```python
from build123d import *
from OCP.BRepFilletAPI import BRepFilletAPI_MakeChamfer

# Parameters (mm, degrees)
SM_BASE_FLANGE_1_DEPTH = 120
CUT_EXTRUDE_1_REACH    = 139.391
SKETCH_6_R             = 1.6
CHAMFER_1_SIZE         = 10
CHAMFER_1_SIZE2        = 50
SKETCH_7_R             = 2.7
CUT_EXTRUDE_2_DEPTH    = 2
SKETCH_9_R             = 2.1
CUT_EXTRUDE_3_DEPTH    = 2
CHAMFER_2_SIZE         = 40
CHAMFER_2_SIZE2        = 15
FILLET_1_R             = 5


# Sheet-metal steps are written as plain solids
with BuildPart() as part:
    # Sketch 1 → 基材-凸緣1 (new body)
    with BuildSketch(Plane.XY):
        with BuildLine():
            Line((-30, 17.5), (-30, -16))
            ThreePointArc((-30, -16), (-29.560660172, -17.060660172), (-28.5, -17.5))
            Line((-28.5, -17.5), (28.5, -17.5))
            ThreePointArc((28.5, -17.5), (29.560660172, -17.060660172), (30, -16))
            Line((30, -16), (30, 17.5))
            Line((30, 17.5), (32, 17.5))
            Line((32, 17.5), (32, -16))
            ThreePointArc((32, -16), (30.974873734, -18.474873734), (28.5, -19.5))
            Line((28.5, -19.5), (-28.5, -19.5))
            ThreePointArc((-28.5, -19.5), (-30.974873734, -18.474873734), (-32, -16))
            Line((-32, -16), (-32, 17.5))
            Line((-32, 17.5), (-30, 17.5))
        make_face()
    extrude(amount=SM_BASE_FLANGE_1_DEPTH)

    # 草圖6 → 除料-伸長1 (cut, up to next)
    with BuildSketch(Plane(origin=(32, 0, 0), x_dir=(0, 0, -1), z_dir=(1, 0, 0)), mode=Mode.PRIVATE) as cut_extrude_1_sk1:
        with Locations(Location((-107.5, 3.5, 0), (0, 0, 90))):
            Circle(SKETCH_6_R)
    cut_extrude_1_tool1 = extrude(cut_extrude_1_sk1.sketch, amount=-CUT_EXTRUDE_1_REACH, mode=Mode.PRIVATE) & part.part
    # 草圖6 → 除料-伸長1 (cut, up to next)
    with BuildSketch(Plane(origin=(32, 0, 0), x_dir=(0, 0, -1), z_dir=(1, 0, 0)), mode=Mode.PRIVATE) as cut_extrude_1_sk2:
        with Locations(Location((-100.5, -3.5, 0), (0, 0, 90))):
            Circle(SKETCH_6_R)
    cut_extrude_1_tool2 = extrude(cut_extrude_1_sk2.sketch, amount=-CUT_EXTRUDE_1_REACH, mode=Mode.PRIVATE) & part.part
    # 草圖6 → 除料-伸長1 (cut, up to next)
    with BuildSketch(Plane(origin=(32, 0, 0), x_dir=(0, 0, -1), z_dir=(1, 0, 0)), mode=Mode.PRIVATE) as cut_extrude_1_sk3:
        with Locations(Location((-107.5, -10.5, 0), (0, 0, 90))):
            Circle(SKETCH_6_R)
    cut_extrude_1_tool3 = extrude(cut_extrude_1_sk3.sketch, amount=-CUT_EXTRUDE_1_REACH, mode=Mode.PRIVATE) & part.part
    # 草圖6 → 除料-伸長1 (cut, up to next)
    with BuildSketch(Plane(origin=(32, 0, 0), x_dir=(0, 0, -1), z_dir=(1, 0, 0)), mode=Mode.PRIVATE) as cut_extrude_1_sk4:
        with Locations(Location((-114.5, -3.5, 0), (0, 0, 90))):
            Circle(SKETCH_6_R)
    cut_extrude_1_tool4 = extrude(cut_extrude_1_sk4.sketch, amount=-CUT_EXTRUDE_1_REACH, mode=Mode.PRIVATE) & part.part
    add(cut_extrude_1_tool1.solids().sort_by_distance((32, 3.5, 107.5))[0], mode=Mode.SUBTRACT)
    add(cut_extrude_1_tool2.solids().sort_by_distance((32, -3.5, 100.5))[0], mode=Mode.SUBTRACT)
    add(cut_extrude_1_tool3.solids().sort_by_distance((32, -10.5, 107.5))[0], mode=Mode.SUBTRACT)
    add(cut_extrude_1_tool4.solids().sort_by_distance((32, -3.5, 114.5))[0], mode=Mode.SUBTRACT)

    # 導角1
    chamfer_1_edges = [part.edges().sort_by_distance(p)[0] for p in [
        (-31, 17.5, 120),
        (31, 17.5, 120),
    ]]
    chamfer_1_side = [part.faces().sort_by_distance(p)[0] for p in [
        (-30.452140533, -17.952140533, 120),
    ]]
    chamfer(chamfer_1_edges, length=CHAMFER_1_SIZE, length2=CHAMFER_1_SIZE2, reference=chamfer_1_side[0])

    # 草圖7 → 除料-伸長2 (cut)
    with BuildSketch(Plane(origin=(32, 0, 0), x_dir=(0, 0, -1), z_dir=(1, 0, 0))):
        with Locations(Location((-107.5, -3.5, 0), (0, 0, 90))):
            Circle(SKETCH_7_R)
    extrude(amount=-CUT_EXTRUDE_2_DEPTH, mode=Mode.SUBTRACT)

    # 草圖9 → 除料-伸長3 (cut)
    with BuildSketch(Plane.ZY.offset(32)):
        with Locations(Location((107.5, -3.5, 0), (0, 0, 270))):
            Circle(SKETCH_9_R)
    extrude(amount=-CUT_EXTRUDE_3_DEPTH, mode=Mode.SUBTRACT)

    # 導角2: one chamfer whose edges measure the first distance from different faces: ONE call of the kernel's chamfer builder (chamfer() names one face for all edges)
    chamfer_2_edges_1 = [part.edges().sort_by_distance(p)[0] for p in [
        (-31, 17.5, 0),
    ]]
    chamfer_2_side_1 = [part.faces().sort_by_distance(p)[0] for p in [
        (-31, 17.5, 35),
    ]]
    chamfer_2_edges_2 = [part.edges().sort_by_distance(p)[0] for p in [
        (31, 17.5, 0),
    ]]
    chamfer_2_side_2 = [part.faces().sort_by_distance(p)[0] for p in [
        (31, 17.5, 35),
    ]]
    chamfer_2 = BRepFilletAPI_MakeChamfer(part.part.solid().wrapped)
    for e in chamfer_2_edges_1:
        chamfer_2.Add(CHAMFER_2_SIZE, CHAMFER_2_SIZE2, e.wrapped, chamfer_2_side_1[0].wrapped)  # the first distance lies on this face
    for e in chamfer_2_edges_2:
        chamfer_2.Add(CHAMFER_2_SIZE, CHAMFER_2_SIZE2, e.wrapped, chamfer_2_side_2[0].wrapped)  # the first distance lies on this face
    add(Compound.cast(chamfer_2.Shape()), mode=Mode.REPLACE)

    # 圓角1
    fillet_1_edges = [part.edges().sort_by_distance(p)[0] for p in [
        (-31, 2.5, 0),
        (31, 2.5, 0),
        (-31, 7.5, 120),
        (31, 7.5, 120),
    ]]
    fillet(fillet_1_edges, radius=FILLET_1_R)


solid = part.part
```
For this review, take the finished solid that the model builds, in its own axes (mm). A direction names the side the tool comes from. Give positions to 0.01 mm unless a question says otherwise; leave off trailing zeros. Write each loop counter-clockwise with the first axis right and the second up, starting at its lowest first coordinate (ties: lowest second). Pieces come first, ordered by that corner, then holes.
Item 1: The part is to be moulded in two halves that separate along X. For faces 1 (the face through (-30.95, -18.5, 59.16)), 2 (the face through (0, -17.5, 59)), 3 (the face through (31, -18.45, 59.16)), say which applies: +X half, -X half, draft (parallel to the pull), parting line (faces both ways), or undercut.
Item 2: Wall thickness on probe 1 along Z at (x, y) = (31.6, -3.5); probe 2 along X at (y, z) = (-5.5, 11.5); probe 3 along Z at (x, y) = (30.8, -10.5): over which ranges is each line inside the solid? List them lowest first.
Item 3: Insertion check: P1, Ø3, axis at x = -21.5, z = 68, coming from the +Y side; P2, Ø5, axis at y = -3.5, z = 107.5, coming from the +X side. Each pin has a flat end and moves straight along its axis. Give the tip position at first contact, or say it passes through.
Item 4: Take a section at D-D (y = -10.5). Give the boundary of the cut face in (x, z), and give its area (3 significant figures).
Item 5: Take a section at C-C (y = -3.5). Give the boundary of the cut face in (x, z).
Item 6: Take a section at B-B (z = 107.5). Give the boundary of the cut face in (x, y), and give its area (3 significant figures).
Item 7: Machinability: for faces 4 (the face through (31.014, 3.292, 109.086)), 5 (the face through (0, -18, 120)), 6 (the face through (-30, -3, 59)), which of the approach directions +Z, -Z, +X, -X, +Y, -Y give a long, thin tool a straight path to every point of the face, cutting with its end or side? Answer none if there is none.
Item 8: Take a section at A-A (y = 10). Give the boundary of the cut face in (x, z), and give its area (3 significant figures).
Established:
1. face 1: -X half
1. face 2: undercut
1. face 3: +X half
2. probe 1: z = 0 to 98.9, 102.1 to 104.8, 110.2 to 112.9, 116.1 to 120
2. probe 2: x = -32 to -30, 30 to 32
2. probe 3: z = 0 to 105.9, 109.1 to 120
3. P1: stops at y = -17.5
3. P2: stops at x = -30
4. outline: (-32, 0) - (-30, 0) - (-30, 120) - (-32, 120) - close; (30, 0) - (32, 0) - (32, 105.9) - (30, 105.9) - close; (30, 109.1) - (32, 109.1) - (32, 120) - (30, 120) - close
4. area: 474 mm2
5. outline: (-32, 0) - (-30, 0) - (-30, 105.4) - (-32, 105.4) - close; (-32, 109.6) - (-30, 109.6) - (-30, 120) - (-32, 120) - close; (30, 0) - (32, 0) - (32, 98.9) - (30, 98.9) - close; (30, 102.1) - (32, 102.1) - (32, 104.8) - (30, 104.8) - close; (30, 110.2) - (32, 110.2) - (32, 112.9) - (30, 112.9) - close; (30, 116.1) - (32, 116.1) - (32, 120) - (30, 120) - close
6. outline: (-32, -16) arc R3.5 ccw to (-28.5, -19.5) - (28.5, -19.5) arc R3.5 ccw to (32, -16) - (32, -12.1) - (30, -12.1) - (30, -16) arc R1.5 cw to (28.5, -17.5) - (-28.5, -17.5) arc R1.5 cw to (-30, -16) - (-30, -5.6) - (-32, -5.6) - close; (-32, -1.4) - (-30, -1.4) - (-30, 10) - (-32, 10) - close; (30, -8.9) - (32, -8.9) - (32, -6.2) - (30, -6.2) - close; (30, -0.8) - (32, -0.8) - (32, 1.9) - (30, 1.9) - close; (30, 5.1) - (32, 5.1) - (32, 10) - (30, 10) - close
6. area: 202 mm2
7. face 4: +X
7. face 5: +Z, +X, -X, +Y, -Y
7. face 6: +Z, -Z, +Y
8. outline: (-32, 20) - (-30, 20) - (-30, 107.5) - (-32, 107.5) - close; (30, 20) - (32, 20) - (32, 107.5) - (30, 107.5) - close
8. area: 350 mm2
